```python
from build123d import *

# Parameters (mm, degrees)
F0_R     = 2.5
F1_DEPTH = 34.6
F2_W     = 1
F2_H     = 3
F2_W_2   = 4.7
F4_W     = 4
F4_H     = 2
F5_DEPTH = 12.5
F6_R     = 0.8
F7_DEPTH = 12.5
F8_SIZE  = 0.5


with BuildPart() as f1:
    # F0 (on Right) → F1 (new body)
    with BuildSketch(Plane.YZ):
        Circle(F0_R)
    extrude(amount=F1_DEPTH)

    # F2 (on Front) → F3 (revolve, cut)
    with BuildSketch(Plane.XZ):
        with Locations((4.7, 3)):
            Rectangle(F2_W, F2_H)
        with Locations((13.25, 3)):
            Rectangle(F2_W_2, F2_H)
        with Locations((22.1, 3)):
            Rectangle(F2_W, F2_H)
    revolve(axis=Axis((18.455703, 0, 0), (1, 0, 0)), mode=Mode.SUBTRACT)

    # F4 (on Front) → F5 (cut, symmetric)
    with BuildSketch(Plane.XZ):
        with Locations((32.6, 0)):
            Rectangle(F4_W, F4_H)
    extrude(amount=F5_DEPTH, both=True, mode=Mode.SUBTRACT)

    # F6 (on Top) → F7 (cut, symmetric)
    with BuildSketch(Plane.XY):
        with Locations((32.6, 0)):
            Circle(F6_R)
    extrude(amount=F7_DEPTH, both=True, mode=Mode.SUBTRACT)

    # F8
    f8_edges = [f1.edges().sort_by_distance(p)[0] for p in [
        (34.6, 0, -2.5),
        (34.6, 0, 2.5),
        (0, -2.5, 0),
    ]]
    chamfer(f8_edges, length=F8_SIZE)


solid = f1.part
```
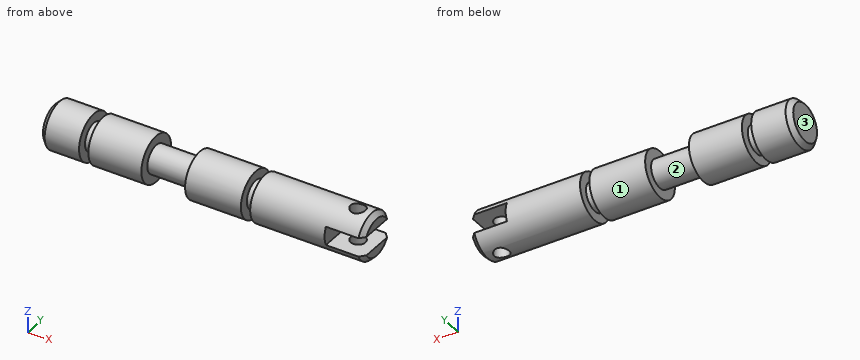
The model under review builds one solid part; all positions refer to its coordinate system, in mm. Face numbers are marked on the shaded views. Coordinates: 2 decimals unless noted, no trailing zeros. Loops run counter-clockwise (first coordinate to the right, second up) from the corner with the lowest first, then second, coordinate; pieces in that order, holes last. Notation, with made-up numbers: (39, -0.75) -> (68, -0.75) arc R21 cw to (68, 28.25) -> close; hole circle Ø10 at (86, 6.25). An arc over 180 degrees is marked (long way). Answer as CSV lines item,"result".
Item 1: Draft analysis for pull direction X (two halves, no side actions). For the marked faces 1, 2 and 3, state which applies: +X half, -X half, draft (parallel to the pull), parting line (faces both ways), or undercut.
Results below:
face 1,"draft"
face 2,"undercut"
face 3,"-X half"
Item 2: For L1, parallel to X at y = 0, z = -1.6; L2, parallel to X at y = 1.85, z = -0.25; L3, parallel to X at y = 0, z = -2.2, list the stretches that pass through material, from the lowest coordinate up.
Results below:
L1,"x = 0 to 4.2, 5.2 to 10.9, 15.6 to 21.6, 22.6 to 31.8, 33.4 to 34.6"
L2,"x = 0 to 4.2, 5.2 to 10.9, 15.6 to 21.6, 22.6 to 30.6"
L3,"x = 0.2 to 4.2, 5.2 to 10.9, 15.6 to 21.6, 22.6 to 31.8, 33.4 to 34.4"
Item 3: Insertion check: pin 1 (1.5 mm diameter, centred on x = 13, y = -0.5, fed in from -Z); pin 2 (1 mm diameter, centred on x = 11.5, z = 0.5, fed in from -Y); pin 3 (1.5 mm diameter, centred on y = 0, z = 1, fed in from -X); pin 4 (1 mm diameter, centred on x = 18, z = -1, fed in from -Y). Each pin has a flat end and moves straight along its axis. Give the tip position at first contact, or say it passes through.
Results below:
pin 1,"stops at z = -1.5"
pin 2,"stops at y = -1.5"
pin 3,"stops at x = 0"
pin 4,"stops at y = -2.45"
Item 4: Take a section at C-C, the plane y = 0. Count the separate pieces of the cut face and the enclosed holes in it, and give its area (3 significant figures).
Results below:
separate pieces,"3"
enclosed holes,"0"
area,"146 mm2"
Item 5: Take a section at D-D, the plane x = 16. State the section outline as (y, z) points.
Results below:
outline,"circle Ø5 at (0, 0)"
Item 6: Take a section at A-A, the plane x = 32.6. State the section outline as (y, z) points, and give its area (3 significant figures).
Results below:
outline,"(-2.29, -1) arc R2.5 ccw to (-0.8, -2.37) -> (-0.8, -1) -> close; (-2.29, 1) -> (-0.8, 1) -> (-0.8, 2.37) arc R2.5 ccw to start; (0.8, -2.37) arc R2.5 ccw to (2.29, -1) -> (0.8, -1) -> close; (0.8, 1) -> (2.29, 1) arc R2.5 ccw to (0.8, 2.37) -> close"
area,"5.25 mm2"
